from build123d import *

# Parameters (mm, degrees)
F1_DEPTH = 2
F3_DEPTH = 6
F4_W     = 15
F4_H     = 3
F5_DEPTH = 15
F6_R     = 2.25
F7_DEPTH = 3.001
F8_R     = 5


with BuildPart() as f1:
    # F0 (on Right) → F1 (new body)
    with BuildSketch(Plane.YZ):
        with BuildLine():
            Line((-28, 25.75), (-28, 0))
            Line((-28, 0), (28, 0))
            Line((28, 0), (28, 25.75))
            ThreePointArc((28, 25.75), (19.872213, 45.372213), (0.25, 53.5))
            Line((0.25, 53.5), (-0.25, 53.5))
            ThreePointArc((-0.25, 53.5), (-19.872213, 45.372213), (-28, 25.75))
        make_face()
    extrude(amount=F1_DEPTH)

    # F2 (on face) → F3 (join)
    with BuildSketch(Plane(origin=(0, 0, 0), x_dir=(0, -1, 0), z_dir=(-1, 0, 0))):
        with BuildLine():
            ThreePointArc((0.25, 51.5), (18.458, 43.958), (26, 25.75))
            Line((26, 25.75), (26, 0))
            Line((26, 0), (28, 0))
            Line((28, 0), (28, 25.75))
            ThreePointArc((28, 25.75), (19.872213, 45.372213), (0.25, 53.5))
            Line((0.25, 53.5), (-0.25, 53.5))
            ThreePointArc((-0.25, 53.5), (-19.872213, 45.372213), (-28, 25.75))
            Line((-28, 25.75), (-28, 0))
            Line((-28, 0), (-26, 0))
            Line((-26, 0), (-26, 25.75))
            ThreePointArc((-26, 25.75), (-18.458, 43.958), (-0.25, 51.5))
            Line((-0.25, 51.5), (0.25, 51.5))
        make_face()
    extrude(amount=F3_DEPTH)

    # F4 (on face) → F5 (join)
    with BuildSketch(Plane(origin=(0, 0, 0), x_dir=(0, -1, 0), z_dir=(-1, 0, 0))):
        with Locations((-20.5, 1.5)):
            Rectangle(F4_W, F4_H)
        with Locations((20.5, 1.5)):
            Rectangle(F4_W, F4_H)
    extrude(amount=F5_DEPTH)

    # F6 (on face) → F7 (cut, through all)
    with BuildSketch(Plane.XY.offset(3)):
        with Locations((-10, 23)):
            Circle(F6_R)
        with Locations((-10, -23)):
            Circle(F6_R)
    extrude(amount=-F7_DEPTH, mode=Mode.SUBTRACT)

    # F8
    f8_edges = [f1.edges().sort_by_distance(p)[0] for p in [
        (-15, 28, 1.5),
        (-15, 13, 1.5),
        (-15, -13, 1.5),
        (-15, -28, 1.5),
    ]]
    fillet(f8_edges, radius=F8_R)


solid = f1.part
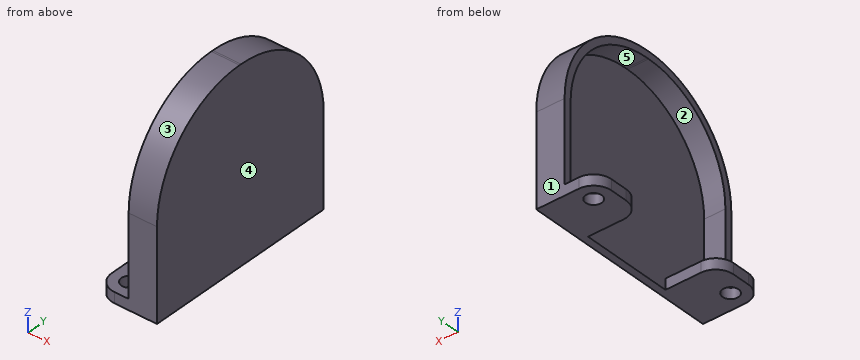
CAD build for the part. Positions are in the model's coordinates, mm. Face numbers are marked on the shaded views. A direction names the side the tool comes from. Coordinates: 2 decimals unless noted, no trailing zeros. Write each loop counter-clockwise with the first axis right and the second up, starting at its lowest first coordinate (ties: lowest second). Pieces come first, ordered by that corner, then holes. Notation, with made-up numbers: M 1.5,22.5 L 7.5,22.5 A18 ccw 7.5,40.5 Z; hole C 74,59.25 d1. An arc over 180 degrees is marked long. Return JSON: item names as keys, results as strings.
Item 1: Slice it at C-C, the plane x = -1.75. Write the cut outline in (y, z), and give its area (3 significant figures).
Findings below:
{"outline": "M -28,0 L -13,0 L -13,3 L -26,3 L -26,25.75 A25.75 cw -0.25,51.5 L 0.25,51.5 A25.75 cw 26,25.75 L 26,3 L 13,3 L 13,0 L 28,0 L 28,25.75 A27.75 ccw 0.25,53.5 L -0.25,53.5 A27.75 ccw -28,25.75 Z", "area": "350 mm2"}
Item 2: Two-plate mould, pull along Z, no slides. Class the marked faces 3, 4 and 5: +Z half, -Z half, draft (parallel to the pull), parting line (faces both ways), or undercut.
Findings below:
{"face 3": "+Z half", "face 4": "draft", "face 5": "undercut"}
Item 3: Slice it at B-B, the plane x = -10.75. Write the cut outline in (y, z).
Findings below:
{"outline": "M -27.94,0 L -25.12,0 L -25.12,3 L -27.94,3 Z; M -20.88,0 L -13.06,0 L -13.06,3 L -20.88,3 Z; M 13.06,0 L 20.88,0 L 20.88,3 L 13.06,3 Z; M 25.12,0 L 27.94,0 L 27.94,3 L 25.12,3 Z"}
Item 4: Probe line 1 (Y direction, x = -10, z = 1.55); line 2 (Z direction, x = -7, y = 24.5); line 3 (Z direction, x = -4, y = -17). List the from-to ranges inside material, lowest first. Write a range as from..to.
Findings below:
{"line 1": "y = -28..-25.25, -20.75..-13, 13..20.75, 25.25..28", "line 2": "z = 0..3", "line 3": "z = 0..3, 45.31..47.87"}
Item 5: Slice it at D-D, the plane y = 2. Write the cut outline in (x, z).
Findings below:
{"outline": "M -6,51.44 L 0,51.44 L 0,0 L 2,0 L 2,53.44 L -6,53.44 Z"}
Item 6: Drop flat-ended pins along their axis: pin 1 Ø4 at (x, y) = (-10, -23) entering from +Z; pin 2 Ø6 at (y, z) = (17.5, 37) entering from -X; pin 3 Ø10 at (x, y) = (-10, -15) entering from +Z; pin 4 Ø10 at (x, y) = (-4.5, -10) entering from -Z. Give the stop position or say it passes through.
Findings below:
{"pin 1": "passes through", "pin 2": "stops at x = 0", "pin 3": "stops at z = 50.89", "pin 4": "stops at z = 0"}
Item 7: Slice it at A-A, the plane z = 20. Write the cut outline in (x, y).
Findings below:
{"outline": "M -6,-28 L 2,-28 L 2,28 L -6,28 L -6,26 L 0,26 L 0,-26 L -6,-26 Z"}
Item 8: Which spindle directions (+Z, -Z, +X, -X, +Y, -Y) get a long thin tool onto all of the face, cutting with end or side? Do the marked faces 1 and 2. Say none if no direction does.
Findings below:
{"face 1": "+Z, -Z, +X, -X, +Y", "face 2": "-X"}
